Could you check a few things on this model? Use its own coordinates, in mm. A direction names the side the tool comes from. Give positions to 0.01 mm unless a question says otherwise; leave off trailing zeros. Order: outer loops, then holes, each group sorted by start corner. A loop starts at its lowest first (then second) coordinate and runs counter-clockwise, first axis right, second up. Notation, with made-up numbers: (87, -26.5) -> (146, -26.5) arc R19 cw to (146, -6.5) -> close; hole circle Ø5 at (84, -31.75). An arc over 180 degrees is marked (long way). One line per item, written item: value.
```python
from build123d import *

# Parameters (mm, degrees)
SKETCH1_W           = 67
SKETCH1_H           = 17.2
BOSS_EXTRUDE1_DEPTH = 2.6
SKETCH2_R           = 1.5
CUT_EXTRUDE1_DEPTH  = 2.6
SKETCH3_W           = 3.782264846
SKETCH3_H           = 4.781353673
BOSS_EXTRUDE2_DEPTH = 1.6


with BuildPart() as part:
    # Sketch1 → Boss-Extrude1 (new body)
    with BuildSketch(Plane(origin=(0, 0, 0), x_dir=(1, 0, 0), z_dir=(0, 1, 0))):
        Rectangle(SKETCH1_W, SKETCH1_H)
    extrude(amount=BOSS_EXTRUDE1_DEPTH)

    # Sketch2 → Cut-Extrude1 (cut)
    with BuildSketch(Plane(origin=(0, 2.6, 0), x_dir=(1, 0, 0), z_dir=(0, 1, 0))):
        with Locations(Location((-18.65, -4.75, 0), (0, 0, 270))):
            Circle(SKETCH2_R)
        with Locations(Location((18.65, -4.75, 0), (0, 0, 270))):
            Circle(SKETCH2_R)
    extrude(amount=-CUT_EXTRUDE1_DEPTH, mode=Mode.SUBTRACT)

    # Sketch3 → Boss-Extrude2 (add)
    with BuildSketch(Plane(origin=(0, 2.6, 0), x_dir=(1, 0, 0), z_dir=(0, 1, 0))):
        with Locations((-20.894711683, 3.782264846)):
            Rectangle(SKETCH3_W, SKETCH3_H)
        with Locations((-29.294711683, 3.782264846)):
            Rectangle(SKETCH3_W, SKETCH3_H)
        with Locations((-12.494711683, 3.782264846)):
            Rectangle(SKETCH3_W, SKETCH3_H)
        with Locations((-4.094711683, 3.782264846)):
            Rectangle(SKETCH3_W, SKETCH3_H)
        with Locations((4.305288317, 3.782264846)):
            Rectangle(SKETCH3_W, SKETCH3_H)
        with Locations((12.705288317, 3.782264846)):
            Rectangle(SKETCH3_W, SKETCH3_H)
        with Locations((21.105288317, 3.782264846)):
            Rectangle(SKETCH3_W, SKETCH3_H)
        with Locations((29.505288317, 3.782264846)):
            Rectangle(SKETCH3_W, SKETCH3_H)
    extrude(amount=BOSS_EXTRUDE2_DEPTH)


solid = part.part
```
1) Suppose I cut it at D-D, the plane x = -8. Write out the boundary of the cut face in (y, z), then the cut area to 3 significant figures.
Answer below:
outline: (0, -8.6) -> (2.6, -8.6) -> (2.6, 8.6) -> (0, 8.6) -> close
area: 44.7 mm2
2) For faces 1 (the flat face through (-4, 3, -6.173)), 2 (the flat face through (-5.986, 3, -4)), 3 (the cylindrical face through (19.915, 1.318, 5.556)), 4 (the flat face through (-13, 3, -1.392)), which set-ups out of +Z, -Z, +X, -X, +Y, -Y let a thin tool reach every point of the face, with its end or its side?
Answer below:
face 1: -Z, +X, -X, +Y
face 2: +Z, -Z, +Y
face 3: +Y, -Y
face 4: +Z, +X, -X, +Y
3) Suppose I cut it at B-B, the plane x = 18.65. Write out the boundary of the cut face in (y, z), then the cut area to 3 significant figures.
Answer below:
outline: (0, -8.6) -> (2.6, -8.6) -> (2.6, 3.25) -> (0, 3.25) -> close; (0, 6.25) -> (2.6, 6.25) -> (2.6, 8.6) -> (0, 8.6) -> close
area: 36.9 mm2
4) We'd pull the mould along X, two halves only. Please class faces 5 (the flat face through (33.5, 1, 0)), 6 (the flat face through (27.614, 3, -4)), 7 (the flat face through (-31.186, 3, -4)), 8 (the flat face through (29, 3, -6.173)): +X half, -X half, draft (parallel to the pull), parting line (faces both ways), or undercut.
Answer below:
face 5: +X half
face 6: undercut
face 7: -X half
face 8: draft
5) If I drill on line 1 along X through (y, z) = (1.55, 4.75); line 2 along X through (y, z) = (1.8, 5.75); line 3 along Y through (x, z) = (-3, 7.5), over which ranges is the centre line in solid material (lowest first)?
Answer below:
line 1: x = -33.5 to -20.15, -17.15 to 17.15, 20.15 to 33.5
line 2: x = -33.5 to -19.77, -17.53 to 17.53, 19.77 to 33.5
line 3: y = 0 to 2.6
6) Suppose I cut it at A-A, the plane z = 4.75. Write out the boundary of the cut face in (x, y).
Answer below:
outline: (-33.5, 0) -> (-20.15, 0) -> (-20.15, 2.6) -> (-33.5, 2.6) -> close; (-17.15, 0) -> (17.15, 0) -> (17.15, 2.6) -> (-17.15, 2.6) -> close; (20.15, 0) -> (33.5, 0) -> (33.5, 2.6) -> (20.15, 2.6) -> close
7) For P1, Ø0.8, axis at y = 3.5, z = -3, coming from the +X side; P2, Ø0.5, axis at x = 3.5, y = 3, coming from the +Z side; P3, Ø1.3, axis at y = 3, z = -4, coming from the -X side; P4, Ø1.3, axis at y = 3.5, z = -4.5, coming from the -X side, each with a flat end and sliding along its axis, tell me the tip position at first contact or that it passes through.
Answer below:
P1: stops at x = 31.4
P2: stops at z = -1.39
P3: stops at x = -33.5
P4: stops at x = -31.19
8) Suppose I cut it at C-C, the plane y = 3.55. State how many separate pieces and enclosed holes the cut face has, then the cut area to 3 significant figures.
Answer below:
separate pieces: 8
enclosed holes: 0
area: 145 mm2
